Answer from the drawing. Dimensions are ordinates in mm from the lowest x, y and z of the part. A direction names the side the tool comes from. Round coordinates to 2 decimals unless told otherwise and drop trailing zeros. Order: outer loops, then holes, each group sorted by start corner. A loop starts at its lowest first (then second) coordinate and runs counter-clockwise, first axis right, second up.
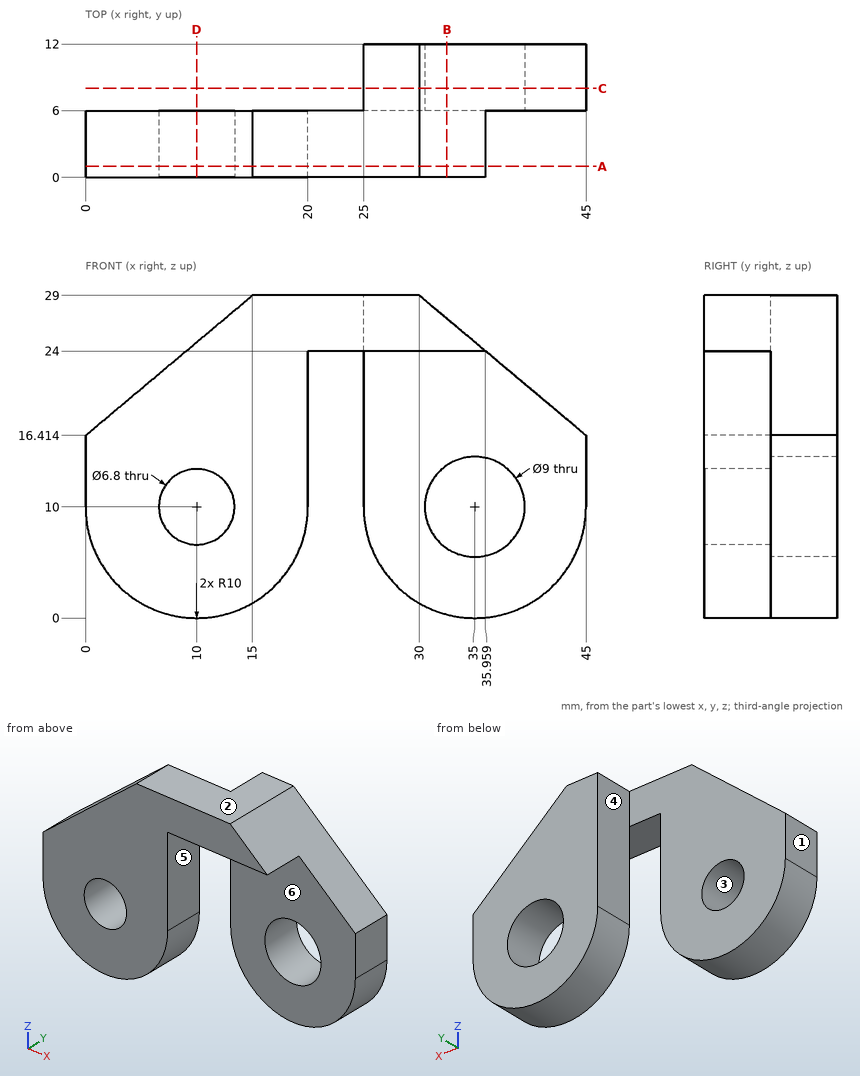
Q1. A cutting plane is placed at C-C, the plane y = 8. Give the vertices of the cut face in (x, z), plus the area to 3 significant figures.
Outcome:
outline: (25, 10) arc R10 ccw to (45, 10) - (45, 16.41) - (30, 29) - (25, 29) - close; hole circle Ø9 at (35, 10)
area: 379 mm2
Q2. A cutting plane is placed at B-B, the plane x = 32.5. Give the vertices of the cut face in (y, z).
Outcome:
outline: (0, 24) - (6, 24) - (6, 13.74) - (12, 13.74) - (12, 26.9) - (0, 26.9) - close; (6, 0.32) - (12, 0.32) - (12, 6.26) - (6, 6.26) - close
Q3. For a pull along X with two mould halves and no side action, classify the marked faces 1, 2 and 3 as released by +X, released by -X, zero draft, split by the parting line, or undercut.
Outcome:
face 1: released by -X
face 2: zero draft
face 3: undercut
Q4. Straight lines are drawn through the part: probe 1 along Y at (x, z) = (9, 22.25); probe 2 along Z at (x, y) = (21, 2); probe 3 along Z at (x, y) = (35, 9.5) (1 decimal). For each, find the intervals that lie inside material, in ascending order.
Outcome:
probe 1: y = 0 to 6
probe 2: z = 24 to 29
probe 3: z = 0 to 5.5, 14.5 to 24.8
Q5. A cutting plane is placed at D-D, the plane x = 10. Give the vertices of the cut face in (y, z) (1 decimal), plus the area to 3 significant figures.
Outcome:
outline: (0, 0) - (6, 0) - (6, 6.6) - (0, 6.6) - close; (0, 13.4) - (6, 13.4) - (6, 24.8) - (0, 24.8) - close
area: 108 mm2
Q6. Flat-ended cylindrical pins translate along their axes: pin 1 (6.5 mm diameter, centred on y = 8.5, z = 22, fed in from -X) (1 decimal); pin 2 (3 mm diameter, centred on y = 3, z = 19, fed in from +X); pin 3 (9 mm diameter, centred on x = 10, z = 10, fed in from +Y). Find the tip coordinate at first contact, or state that the pin passes through.
Outcome:
pin 1: stops at x = 4.2
pin 2: stops at x = 20
pin 3: stops at y = 6
Q7. A cutting plane is placed at A-A, the plane y = 1. Give the vertices of the cut face in (x, z).
Outcome:
outline: (0, 10) arc R10 ccw to (20, 10) - (20, 24) - (35.96, 24) - (30, 29) - (15, 29) - (0, 16.41) - close; hole circle Ø6.8 at (10, 10)
Q8. For the marked faces 4, 5 and 6, determine the directions among +Z, -Z, +X, -X, +Y, -Y from which every point of the face is accessible in a straight line to the end or side of a thin tool.
Outcome:
face 4: +Z, -Z, -X, +Y
face 5: -Z, +X, +Y, -Y
face 6: -Z, +X, -Y
